Model file for the job. Use its own axes, mm. A direction names the side the tool comes from. Round coordinates to 2 decimals unless told otherwise and drop trailing zeros. Write each loop counter-clockwise with the first axis right and the second up, starting at its lowest first coordinate (ties: lowest second). Pieces come first, ordered by that corner, then holes. Notation, with made-up numbers: (-7, 2.25) - (6, 2.25) arc R18 ccw to (6, 23.25) - close; hole circle Ø7 at (38, 69.25). An arc over 180 degrees is marked (long way). Answer as a JSON object with one key per item and string values. Group by question number.
from build123d import *

# Parameters (mm, degrees)
BOSS_EXTRUDE1_DEPTH      = 8
BOSS_EXTRUDE2_DEPTH      = 5
BOSS_EXTRUDE2_DEPTH_BACK = 5
SKETCH3_R                = 10
BOSS_EXTRUDE3_DEPTH      = 12.9
BOSS_EXTRUDE3_DEPTH_BACK = 12.9
SKETCH4_W                = 3.3
SKETCH4_H                = 8
SKETCH5_W                = 3.3
SKETCH5_H                = 8
SKETCH6_W                = 3.3
SKETCH6_H                = 8
SKETCH7_W                = 3.3
SKETCH7_H                = 8


with BuildPart() as part:
    # Sketch1 → Boss-Extrude1 (new body)
    with BuildSketch(Plane(origin=(0, 0, 0), x_dir=(1, 0, 0), z_dir=(0, 1, 0))):
        with BuildLine():
            Line((-19.5, -15.5), (19.5, -15.5))
            ThreePointArc((19.5, -15.5), (23.742640687, -13.742640687), (25.5, -9.5))
            Line((25.5, -9.5), (25.5, 9.5))
            ThreePointArc((25.5, 9.5), (23.742640687, 13.742640687), (19.5, 15.5))
            Line((19.5, 15.5), (-19.5, 15.5))
            ThreePointArc((-19.5, 15.5), (-23.742640687, 13.742640687), (-25.5, 9.5))
            Line((-25.5, 9.5), (-25.5, -9.5))
            ThreePointArc((-25.5, -9.5), (-23.742640687, -13.742640687), (-19.5, -15.5))
        make_face()
    extrude(amount=BOSS_EXTRUDE1_DEPTH)

    # Sketch2 → Boss-Extrude2 (add, two sides)
    with BuildSketch(Plane(origin=(0, 0, 0), x_dir=(0, 0, -1), z_dir=(1, 0, 0))) as boss_extrude2_sk:
        Polygon((-21.265544457, 29.517304845), (-15.5, 8), (13.585782237, 8), (-3.482172222, 34.282345074), align=None)
    extrude(amount=BOSS_EXTRUDE2_DEPTH)
    extrude(boss_extrude2_sk.sketch, amount=-BOSS_EXTRUDE2_DEPTH_BACK)

    # Sketch3 → Boss-Extrude3 (add, two sides)
    with BuildSketch(Plane(origin=(0, 0, 0), x_dir=(0, 0, -1), z_dir=(1, 0, 0))) as boss_extrude3_sk:
        with Locations((-12, 32)):
            Circle(SKETCH3_R)
    extrude(amount=BOSS_EXTRUDE3_DEPTH)
    extrude(boss_extrude3_sk.sketch, amount=-BOSS_EXTRUDE3_DEPTH_BACK)

    # Sketch4 → Cut-Revolve1 (revolve, cut)
    with BuildSketch(Plane.XY.offset(9)):
        with Locations((-20.65, 4)):
            Rectangle(SKETCH4_W, SKETCH4_H)
    revolve(axis=Axis((-19, 8, 9), (0, -1, 0)), mode=Mode.SUBTRACT)

    # Sketch5 → Cut-Revolve2 (revolve, cut)
    with BuildSketch(Plane.XY.offset(9)):
        with Locations((17.35, 4)):
            Rectangle(SKETCH5_W, SKETCH5_H)
    revolve(axis=Axis((19, 8, 9), (0, -1, 0)), mode=Mode.SUBTRACT)

    # Sketch6 → Cut-Revolve3 (revolve, cut)
    with BuildSketch(Plane.XY.offset(-9)):
        with Locations((-20.65, 4)):
            Rectangle(SKETCH6_W, SKETCH6_H)
    revolve(axis=Axis((-19, 8, -9), (0, -1, 0)), mode=Mode.SUBTRACT)

    # Sketch7 → Cut-Revolve4 (revolve, cut)
    with BuildSketch(Plane.XY.offset(-9)):
        with Locations((17.35, 4)):
            Rectangle(SKETCH7_W, SKETCH7_H)
    revolve(axis=Axis((19, 8, -9), (0, -1, 0)), mode=Mode.SUBTRACT)

    # Sketch8 → Cut-Revolve5 (revolve, cut)
    with BuildSketch(Plane.XY.offset(12)):
        Polygon((-12.9, 32), (-12.9, 39.5), (-12.611324865, 39), (12.611324865, 39), (12.9, 39.5), (12.9, 32), align=None)
    revolve(axis=Axis((12.9, 32, 12), (-1, 0, 0)), mode=Mode.SUBTRACT)

    # Sketch9 → Revolve1 (revolve)
    with BuildSketch(Plane.XY.offset(12)):
        Polygon((-12.9, 37.3), (-12.6, 37), (12.6, 37), (12.9, 37.3), (12.9, 38.7), (12.6, 39), (-12.6, 39), (-12.9, 38.7), align=None)
    revolve(axis=Axis((12.9, 32, 12), (-1, 0, 0)))


solid = part.part
(1) Slice it at D-D (y = 19.5). Write the cut outline in (x, z), then the cut area to 3 significant figures.
(2) Slice it at B-B (x = 18.5). Write the cut outline in (y, z).
(3) 3-axis set-ups, long thin cutter, end or side, ignore diameter. For faces 1 (the flat face through (-12.9, 32.5, 6.5)), 2 (the flat face through (0.07, 19.832, -5.902)): which of +Z, -Z, +X, -X, +Y, -Y reach the whole face in a straight line?
(4) Slice it at A-A (x = -4). Write the cut outline in (y, z).
(5) Pull direction Y, two halves, no side cores. Call faces 3 (the flat face through (5.3, 8, -0.2)), 4 (the flat face through (-12.9, 39, 8)), 5 (the flat face through (0.07, 17.525, 18.052)): pulls with the +Y half, pulls with the -Y half, needs draft (parallel to the pull), parting line crosses it, or undercut.
(6) Slice it at C-C (z = -1). Write the cut outline in (x, y).
(7) Flat gauge pins, fed straight in: pin 1 (4 mm diameter, centred on x = 2, y = 4.5, fed in from +Z); pin 2 (14.5 mm diameter, centred on y = 33, z = 15.5, fed in from +X); pin 3 (14.5 mm diameter, centred on y = 35, z = 11, fed in from -X). Where does each tip first touch, or does it go through?
(8) Drill centre lines: line 1 (X direction, y = 2.75, z = 9); line 2 (Z direction, x = -19, y = 2.5); line 3 (Y direction, x = -11, z = 8.5). Where is each one in solid material? Low to high. Write a range as from..to.
Answer:
{
 "1": {"outline": "(-5, -6.12) - (5, -6.12) - (5, 18.58) - (-5, 18.58) - close", "area": "247 mm²"},
 "2": {"outline": "(0, -15.5) - (8, -15.5) - (8, -12.26) - (0, -12.26) - close; (0, -5.74) - (8, -5.74) - (8, 5.74) - (0, 5.74) - close; (0, 12.26) - (8, 12.26) - (8, 15.5) - (0, 15.5) - close"},
 "3": {"face 1": "+Z, -Z, -X, +Y", "face 2": "-Z, +X, -X, +Y"},
 "4": {"outline": "(0, -15.5) - (8, -15.5) - (8, -13.59) - (32, 2) arc R10 ccw (long way) to (26.79, 20.53) - (8, 15.5) - (0, 15.5) - close; hole circle Ø10 at (32, 12)"},
 "5": {"face 3": "undercut", "face 4": "needs draft", "face 5": "pulls with the -Y half"},
 "6": {"outline": "(-25.5, 0) - (25.5, 0) - (25.5, 8) - (5, 8) - (5, 27.38) - (-5, 27.38) - (-5, 8) - (-25.5, 8) - close"},
 "7": {"pin 1": "z = 15.5", "pin 2": "x = 12.9", "pin 3": "x = -12.9"},
 "8": {"line 1": "-25.5..-22.3, -15.7..15.7, 22.3..25.5", "line 2": "-15.5..-12.3, -5.7..5.7, 12.3..15.5", "line 3": "0..8, 22.63..28.43, 35.57..41.37"}
}
